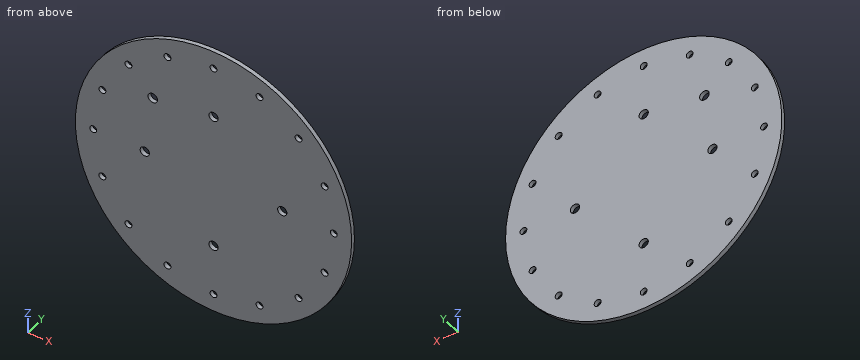
from build123d import *

# Parameters (mm, degrees)
F0_R     = 160.8
F1_DEPTH = 4.763
F3_D     = 10.75
F5_D     = 8
F7_D     = 11.1


with BuildPart() as f1:
    # F0 (on Front) → F1 (new body)
    with BuildSketch(Plane.XZ):
        Circle(F0_R)
    extrude(amount=F1_DEPTH)

    # F3 (through all)
    with Locations(Plane.XZ.offset(4.763)):
        with Locations((-80, 0), (0, 80), (80, 0), (0, -80)):
            Hole(F3_D / 2)

    # F5 (through all)
    with Locations(Plane.XZ.offset(4.763)):
        with Locations((-53.575681, 129.343135), (0, 140), (53.575681, 129.343135), (98.994949, 98.994949), (129.343135, 53.575681), (140, 0), (129.343135, -53.575681), (98.994949, -98.994949), (53.575681, -129.343135), (0, -140), (-53.575681, -129.343135), (-98.994949, -98.994949), (-129.343135, -53.575681), (-140, 0), (-129.343135, 53.575681), (-98.994949, 98.994949)):
            Hole(F5_D / 2)

    # F7 (through all)
    with Locations(Plane.XZ.offset(4.763)):
        with Locations((-70.710678, 70.710678)):
            Hole(F7_D / 2)


solid = f1.part
Check sheet for the modelled part. Datum: model origin and axes. Units: mm. Give positions to 0.01 mm unless a question says otherwise; leave off trailing zeros. Loops run counter-clockwise (first coordinate to the right, second up) from the corner with the lowest first, then second, coordinate; pieces in that order, holes last. Notation, with made-up numbers: M 61.5,-38.75 L 71.5,-38.75 A13 ccw 71.5,-22.75 Z; hole C 13.25,21 d4. An arc over 180 degrees is marked long. Use a Markdown table: item, result. Add a question column.
Q1. Sectioned sample at B-B, the plane z = 0. Record the cut outline in (x, y) (3 decimals), then the cut area to 3 significant figures.
Q2. Scan lines: line 1 along Z through (x, y) = (0, -1.55) (3 decimals); line 2 along X through (y, z) = (-4.35, 133) (3 decimals); line 3 along Z through (x, y) = (99.5, -2.25). Record each from-to range of solid material in increasing order. Write a range as [from, to].
Q3. Go/stop test with flat-tipped pins: pin 1 (9 mm diameter, centred on x = -53.58, z = 129.34, fed in from -Y); pin 2 (1.5 mm diameter, centred on y = -0.5, z = 44.5, fed in from -X); pin 3 (9.5 mm diameter, centred on x = -80, z = 0, fed in from +Y); pin 4 (1.5 mm diameter, centred on x = 9, y = -4, fed in from -Z). Record where each tip stops, or that it passes through.
Q4. Sectioned sample at A-A, the plane x = 0. Record the cut outline in (y, z) (3 decimals), then the cut area to 3 significant figures.
Q5. Sectioned sample at C-C, the plane z = -80. Record the cut outline in (x, y) (3 decimals), then the cut area to 3 significant figures.
Q6. Sectioned sample at D-D, the plane y = -1.5. Give the number of separate pieces and of enclosed holes in the cut face, then the cut area to 3 significant figures.
Verdict:
| question | item | result |
|---|---|---|
| 1 | outline | M -160.8,-4.763 L -144,-4.763 L -144,0 L -160.8,0 Z; M -136,-4.763 L -85.375,-4.763 L -85.375,0 L -136,0 Z; M -74.625,-4.763 L 74.625,-4.763 L 74.625,0 L -74.625,0 Z; M 85.375,-4.763 L 136,-4.763 L 136,0 L 85.375,0 Z; M 144,-4.763 L 160.8,-4.763 L 160.8,0 L 144,0 Z |
| 1 | area | 1,350 mm^2 |
| 2 | line 1 | [-160.8, -144], [-136, -85.375], [-74.625, 74.625], [85.375, 136], [144, 160.8] |
| 2 | line 2 | [-90.375, -55.197], [-51.955, 51.955], [55.197, 90.375] |
| 2 | line 3 | [-126.32, -102.96], [-95.03, 95.03], [102.96, 126.32] |
| 3 | pin 1 | y = -4.76 |
| 3 | pin 2 | x = -154.73 |
| 3 | pin 3 | through |
| 3 | pin 4 | z = -160.59 |
| 4 | outline | M -4.763,-160.8 L 0,-160.8 L 0,-144 L -4.763,-144 Z; M -4.763,-136 L 0,-136 L 0,-85.375 L -4.763,-85.375 Z; M -4.763,-74.625 L 0,-74.625 L 0,74.625 L -4.763,74.625 Z; M -4.763,85.375 L 0,85.375 L 0,136 L -4.763,136 Z; M -4.763,144 L 0,144 L 0,160.8 L -4.763,160.8 Z |
| 4 | area | 1,350 mm^2 |
| 5 | outline | M -139.487,-4.763 L -5.375,-4.763 L -5.375,0 L -139.487,0 Z; M 5.375,-4.763 L 139.487,-4.763 L 139.487,0 L 5.375,0 Z |
| 5 | area | 1,280 mm^2 |
| 6 | separate pieces | 1 |
| 6 | enclosed holes | 21 |
| 6 | area | 80,000 mm^2 |
